from build123d import *

# Parameters (mm, degrees)
F0_R          = 1.5
F0_R_2        = 2.6412895019
F1_DEPTH      = 20
F3_DEPTH      = 25
F3_DEPTH_BACK = 25
F5_DEPTH      = 25
F8_R          = 3
F11_DEPTH     = 20
F12_T1_DEPTH  = 41.4280655281


# Not quite as in the source:
# - a fillet or chamfer that OpenCascade refuses, or shapes differently, is made with other operations: its cross-section is extruded or revolved along the edge and cut away or added


with BuildPart() as f1:
    # F0 (on Top) → F1 (new body)
    with BuildSketch(Plane.XY):
        with BuildLine():
            Line((-136.9092201152, 53.1693232265), (-48.1315898414, 53.1693232265))
            ThreePointArc((-48.1315898414, 53.1693232265), (-24.7040865671, 60.2304450376), (-48.9954501741, 63.1693232265))
            Line((-48.9954501741, 63.1693232265), (-140.1388241649, 63.1693232265))
            Line((-140.1388241649, 63.1693232265), (-164.0276092996, 45.9422132412))
            ThreePointArc((-164.0276092996, 45.9422132412), (-165.0669659453, 38.947333564), (-158.0720862682, 37.9079769183))
            Line((-158.0720862682, 37.9079769183), (-136.9092201152, 53.1693232265))
        make_face()
        with Locations((-161.0498477839, 41.9250950797)):
            Circle(F0_R, mode=Mode.SUBTRACT)
        with BuildLine():
            ThreePointArc((-43.3736355328, 51.5244823211), (-44.7878490952, 51.5244823211), (-44.7878490952, 52.9386958835))
            Line((-44.7878490952, 52.9386958835), (-41.4003457692, 56.3261992095))
            ThreePointArc((-41.4003457692, 56.3261992095), (-39.9861322069, 56.3261992095), (-39.9861322069, 54.9119856471))
            Line((-39.9861322069, 54.9119856471), (-43.3736355328, 51.5244823211))
        make_face(mode=Mode.SUBTRACT)
        with BuildLine():
            ThreePointArc((-29.527561069, 52.9386958835), (-29.527561069, 51.5244823211), (-30.9417746314, 51.5244823211))
            Line((-30.9417746314, 51.5244823211), (-34.3292779574, 54.9119856471))
            ThreePointArc((-34.3292779574, 54.9119856471), (-34.3292779574, 56.3261992095), (-32.915064395, 56.3261992095))
            Line((-32.915064395, 56.3261992095), (-29.527561069, 52.9386958835))
        make_face(mode=Mode.SUBTRACT)
        with Locations((-37.1577050821, 59.1546263342)):
            Circle(F0_R_2, mode=Mode.SUBTRACT)
        with BuildLine():
            Line((-41.4003457692, 61.9830534589), (-44.7878490952, 65.3705567849))
            ThreePointArc((-44.7878490952, 65.3705567849), (-44.7878490952, 66.7847703473), (-43.3736355328, 66.7847703473))
            Line((-43.3736355328, 66.7847703473), (-39.9861322069, 63.3972670213))
            ThreePointArc((-39.9861322069, 63.3972670213), (-39.9861322069, 61.9830534589), (-41.4003457692, 61.9830534589))
        make_face(mode=Mode.SUBTRACT)
        with BuildLine():
            ThreePointArc((-30.9417746314, 66.7847703473), (-29.527561069, 66.7847703473), (-29.527561069, 65.3705567849))
            Line((-29.527561069, 65.3705567849), (-32.915064395, 61.9830534589))
            ThreePointArc((-32.915064395, 61.9830534589), (-34.3292779574, 61.9830534589), (-34.3292779574, 63.3972670213))
            Line((-34.3292779574, 63.3972670213), (-30.9417746314, 66.7847703473))
        make_face(mode=Mode.SUBTRACT)
    extrude(amount=F1_DEPTH)

    # F2 (on face) → F3 (cut, two sides)
    with BuildSketch(Plane.XZ.offset(-53.1693232265)) as f3_sk:
        with BuildLine():
            add(Edge.make_bspline(
                [(-48.1315898414, 5.1997262053), (-55.5737955735, 5.517366778), (-70.0693075174, 9.5402547737), (-82.2478533544, 13.4277092293)],
                knots=[0, 0, 0, 0, 32.5655157772, 32.5655157772, 32.5655157772, 32.5655157772], degree=3))
            Line((-48.1315898414, 5.1997262053), (-22.6805435396, 5.1997262053))
            Line((-22.6805435396, 5.1997262053), (-24.4416198375, 23.0218202323))
            Line((-24.4416198375, 23.0218202323), (-102.9450073838, 23.9689107984))
            Line((-102.9450073838, 23.9689107984), (-109.8586171865, 20))
            Line((-109.8586171865, 20), (-136.9092201152, 24.3437178433))
            Line((-136.9092201152, 24.3437178433), (-136.9092201152, 13.4277092293))
            Line((-136.9092201152, 13.4277092293), (-82.2478533544, 13.4277092293))
        make_face()
    extrude(amount=-F3_DEPTH, mode=Mode.SUBTRACT)
    extrude(f3_sk.sketch, amount=F3_DEPTH_BACK, mode=Mode.SUBTRACT)

    # F4 (on face) → F5 (cut)
    with BuildSketch(Plane(origin=(-77.913469167, 108.0423893277, 0), x_dir=(-0.8110964415, -0.5849124402, 0), z_dir=(-0.5849124402, 0.8110964415, 0))):
        with BuildLine():
            Line((73.6283713512, 25.1456971396), (74.0980582459, 13.4277092293))
            add(Edge.make_bspline(
                [(74.0980582459, 13.4277092293), (92.9379910232, 13.834843412), (100.7777675986, 11.1937364563), (101.1828109622, 20)],
                knots=[0, 0, 0, 0, 27.8707523342, 27.8707523342, 27.8707523342, 27.8707523342], degree=3))
            Line((101.1828109622, 20), (97.8787563539, 26.1177145299))
            Line((97.8787563539, 26.1177145299), (73.6283713512, 25.1456971396))
        make_face()
    extrude(amount=-F5_DEPTH, mode=Mode.SUBTRACT)

    # F9: sweep along a path in F6
    with BuildLine(Plane.XY.offset(5.1997262053)) as f9_path:
        Line((-61.2067505717, 58.1693232265), (-86.7135846391, 58.1693232265))
        Line((-86.7135846391, 58.1693232265), (-137.850685735, 58.1693232265))
        Line((-137.850685735, 58.1693232265), (-147.6771980524, 50.9236194193))
        Line((-147.6771980524, 50.9236194193), (-156.9756269455, 10.3533519432))
    # F8 (on face) → F9 (sweep, cut)
    with BuildSketch(Plane.YZ.offset(-48.1315898414)):
        with Locations((58.2011528313, 8.1997262053)):
            Circle(F8_R)
    sweep(path=f9_path.line, transition=Transition.RIGHT, mode=Mode.SUBTRACT)

    # F10 (on face) → F11 (join)
    with BuildSketch(Plane(origin=(0, 0, 0), x_dir=(1, 0, 0), z_dir=(0, 0, -1))):
        Polygon((-159.9824870749, -48.8593044651), (-164.0276092996, -45.9422132412), (-162.4302172451, -52.2535650319), align=None)
    extrude(amount=-F11_DEPTH)

    # F12: fillet of radius 2 on 1 edges, made by hand

    # F12_s2 → F12_t1 (cut)
    with BuildSketch(Plane.XY.offset(-10.7140327641)):
        with BuildLine():
            ThreePointArc((-163.4817415016, 48.0989559734), (-161.9675459982, 49.5626274076), (-159.9824870749, 48.8593044651))
            Line((-159.9824870749, 48.8593044651), (-162.4302172451, 52.2535650319))
            Line((-162.4302172451, 52.2535650319), (-163.4817415016, 48.0989559734))
        make_face()
    extrude(amount=F12_T1_DEPTH, mode=Mode.SUBTRACT)


solid = f1.part
Build history of the part. All positions in model axes, mm. A direction names the side the tool comes from. Round coordinates to 2 decimals unless told otherwise and drop trailing zeros. Loops run counter-clockwise (first coordinate to the right, second up) from the corner with the lowest first, then second, coordinate; pieces in that order, holes last. Notation, with made-up numbers: (8.5, 9) -> (59.5, 9) arc R11 cw to (59.5, 27) -> close; hole circle Ø9 at (18.25, 12.25). An arc over 180 degrees is marked (long way). Answer in a Markdown table with one row per item.
Item 1: Saw through at A-A (x = -37). Write the cut outline in (y, z).
Answers below:
| item | result |
|---|---|
| outline | (46.66, 0) -> (56.52, 0) -> (56.52, 5.2) -> (46.66, 5.2) -> close; (61.79, 0) -> (71.65, 0) -> (71.65, 5.2) -> (61.79, 5.2) -> close |
Item 2: Pin check, flat tips, straight feed: pin 1 (6 mm diameter, centred on y = 54.5, z = 6.5, fed in from +X); pin 2 (8 mm diameter, centred on x = -96, y = 52, fed in from +Z); pin 3 (12 mm diameter, centred on x = -138.5, z = 8, fed in from -Y). Stop position of each tip, or through.
Answers below:
| item | result |
|---|---|
| pin 1 | stops at x = -24.81 |
| pin 2 | stops at z = 13.43 |
| pin 3 | stops at y = 47.7 |
Item 3: Saw through at C-C (x = -104). Write the cut outline in (y, z), and give its area (3 significant figures).
Answers below:
| item | result |
|---|---|
| outline | (53.17, 0) -> (63.17, 0) -> (63.17, 13.43) -> (53.17, 13.43) -> close; hole circle Ø6 at (58.2, 8.2) |
| area | 106 mm² |
Item 4: Drill centre lines: L1, parallel to Y at x = -41.5, z = 4.5; L2, parallel to Z at x = -116.5, y = 53.5; L3, parallel to X at y = 64, z = 3. Where is each one in solid material? Low to high. Write a range as [from, to].
Answers below:
| item | result |
|---|---|
| L1 | y = [47.43, 53.4], [56.23, 62.08], [64.91, 70.88] |
| L2 | z = [0, 13.43] |
| L3 | x = [-48.68, -43.42], [-40.59, -33.73], [-30.9, -25.64] |
Item 5: Which spindle directions (+Z, -Z, +X, -X, +Y, -Y) get a long thin tool onto all of the face, cutting with end or side? Do faces 4 (the flat face through (-37, 62, 5.2)), 5 (the flat face through (-103, 53.169, 7)), 6 (the cylindrical face through (-104.204, 57.811, 5.225)), 7 (the cylindrical face through (-161.998, 49.556, 9.86)), 8 (the flat face through (-32.61, 53.19, 2.56)). Say none if no direction does.
Answers below:
| item | result |
|---|---|
| face 4 | +Z, +X, +Y, -Y |
| face 5 | +Z, -Z, -Y |
| face 6 | +X |
| face 7 | +Z, -Z, +Y |
| face 8 | +Z, -Z |
Item 6: Mould opens along X. For faces 1 (the flat face through (-104, 63.169, 7)), 2 (the flat face through (-31.25, 54.66, 2.56)), 3 (the cylindrical face through (-165.131, 39.036, 9.86)) say: +X half, -X half, draft (parallel to the pull), parting line (faces both ways), or undercut.
Answers below:
| item | result |
|---|---|
| face 1 | draft |
| face 2 | undercut |
| face 3 | parting line |
Item 7: Saw through at B-B (z = 2). Write the cut outline in (x, y).
Answers below:
| item | result |
|---|---|
| outline | (-164.03, 45.94) arc R5 ccw to (-158.07, 37.91) -> (-136.91, 53.17) -> (-48.13, 53.17) arc R12.5 ccw (long way) to (-49, 63.17) -> (-140.14, 63.17) -> (-159.98, 48.86) arc R2 ccw to (-163.48, 48.1) -> close; hole circle Ø3 at (-161.05, 41.93); hole (-44.79, 52.94) arc R1 ccw to (-43.37, 51.52) -> (-39.99, 54.91) arc R1 ccw to (-41.4, 56.33) -> close; hole (-44.79, 65.37) -> (-41.4, 61.98) arc R1 ccw to (-39.99, 63.4) -> (-43.37, 66.78) arc R1 ccw to start; hole circle Ø5.28 at (-37.16, 59.15); hole (-34.33, 54.91) -> (-30.94, 51.52) arc R1 ccw to (-29.53, 52.94) -> (-32.92, 56.33) arc R1 ccw to start; hole (-34.33, 63.4) arc R1 ccw to (-32.92, 61.98) -> (-29.53, 65.37) arc R1 ccw to (-30.94, 66.78) -> close |
